Input: part model. Units: mm. Frame: model coordinates. Coordinates: 2 decimals unless noted, no trailing zeros. Loops run counter-clockwise (first coordinate to the right, second up) from the corner with the lowest first, then second, coordinate; pieces in that order, holes last. Notation, with made-up numbers: (46.5, 37.5) -> (92.5, 37.5) arc R24 ccw to (92.5, 62.5) -> close; hole circle Ø3 at (62, 78). An arc over 180 degrees is marked (long way). Answer as a JSON object with one key per item and string values.
from build123d import *
from OCP.BRepFilletAPI import BRepFilletAPI_MakeChamfer

# Parameters (mm, degrees)
BOSS_EXTRUDE1_DEPTH = 1.3
CUT_EXTRUDE1_DEPTH  = 7.730527468
CUT_EXTRUDE2_DEPTH  = 7.730527468
SKETCH4_W           = 6.4
SKETCH4_H           = 4.4
BOSS_EXTRUDE2_DEPTH = 0.3
SKETCH5_W           = 4.78
SKETCH5_H           = 1.3
BOSS_EXTRUDE3_DEPTH = 0.3
SKETCH6_W           = 4.78
SKETCH6_H           = 1.3
BOSS_EXTRUDE4_DEPTH = 0.3
DRAFT1_ANGLE        = 20
DRAFT2_ANGLE        = 20
HOLE1_D             = 0.497503641
HOLE1_DEPTH         = 0.2
CHAMFER1_SIZE       = 0.234692934
CHAMFER1_SIZE2      = 0.311889554
CHAMFER2_SIZE       = 0.311889554
CHAMFER2_SIZE2      = 0.234692934
FILLET1_R           = 0.5


with BuildPart() as part:
    # Sketch1 → Boss-Extrude1 (new body)
    with BuildSketch(Plane(origin=(0, 1.3, 0), x_dir=(1, 0, 0), z_dir=(0, 1, 0))):
        Polygon((3.5, 2.1), (0, 5.6), (-3.5, 2.1), (-3.5, -2.1), (0, -5.6), (3.5, -2.1), align=None)
    extrude(amount=-BOSS_EXTRUDE1_DEPTH)

    # Sketch2 → Cut-Extrude1 (cut, through all)
    with BuildSketch(Plane.XZ):
        Polygon((0, -5.6), (2.69, -2.91), (2.69, -2.2), (-2.69, -2.2), (-2.69, -2.91), align=None)
    extrude(amount=-CUT_EXTRUDE1_DEPTH, mode=Mode.SUBTRACT)

    # Sketch3 → Cut-Extrude2 (cut, through all)
    with BuildSketch(Plane.XZ):
        Polygon((2.69, 2.2), (2.69, 2.91), (0, 5.6), (-2.69, 2.91), (-2.69, 2.2), align=None)
    extrude(amount=-CUT_EXTRUDE2_DEPTH, mode=Mode.SUBTRACT)

    # Sketch4 → Boss-Extrude2 (add)
    with BuildSketch(Plane(origin=(0, 1.3, 0), x_dir=(-1, 0, 0), z_dir=(0, 1, 0))):
        Rectangle(SKETCH4_W, SKETCH4_H)
    extrude(amount=BOSS_EXTRUDE2_DEPTH)

    # Sketch5 → Boss-Extrude3 (add)
    with BuildSketch(Plane.XY.offset(2.2)):
        with Locations((0, 0.65)):
            Rectangle(SKETCH5_W, SKETCH5_H)
    extrude(amount=BOSS_EXTRUDE3_DEPTH)

    # Sketch6 → Boss-Extrude4 (add)
    with BuildSketch(Plane(origin=(0, 0, -2.2), x_dir=(-1, 0, 0), z_dir=(0, 0, -1))):
        with Locations((0, 0.65)):
            Rectangle(SKETCH6_W, SKETCH6_H)
    extrude(amount=BOSS_EXTRUDE4_DEPTH)

    # Draft1
    draft1_faces = [part.faces().sort_by_distance(p)[0] for p in [
        (-2.69, 0.65, -2.555),
        (-2.39, 0.65, -2.35),
        (2.39, 0.65, -2.35),
        (2.69, 0.65, -2.555),
    ]]
    draft(draft1_faces, Plane(origin=(2.69, 1.3, -2.2), x_dir=(-1, 0, 0), z_dir=(0, 0, -1)), DRAFT1_ANGLE)

    # Draft2
    draft2_faces = [part.faces().sort_by_distance(p)[0] for p in [
        (2.69, 0.65, 2.555),
        (2.39, 0.65, 2.35),
        (-2.39, 0.65, 2.35),
        (-2.69, 0.65, 2.555),
    ]]
    draft(draft2_faces, Plane(origin=(-2.69, 1.3, 2.2), x_dir=(1, 0, 0), z_dir=(0, 0, 1)), DRAFT2_ANGLE)

    # Hole1
    with Locations(Plane(origin=(0, 1.6, 0), x_dir=(1, 0, 0), z_dir=(0, 1, 0))):
        with Locations((-2.524000409, -1.40306368)):
            Hole(HOLE1_D / 2, depth=HOLE1_DEPTH)

    # Chamfer1: one chamfer whose edges measure the first distance from different faces: ONE call of the kernel's chamfer builder (chamfer() names one face for all edges)
    chamfer1_edges_1 = [part.edges().sort_by_distance(p)[0] for p in [
        (-2.879460781, 0.65, -2.720539219),
    ]]
    chamfer1_side_1 = [part.faces().sort_by_distance(p)[0] for p in [
        (-2.784730391, 0.65, -2.460269609),
    ]]
    chamfer1_edges_2 = [part.edges().sort_by_distance(p)[0] for p in [
        (2.879460781, 0.65, 2.720539219),
    ]]
    chamfer1_side_2 = [part.faces().sort_by_distance(p)[0] for p in [
        (2.784730391, 0.65, 2.460269609),
    ]]
    chamfer1 = BRepFilletAPI_MakeChamfer(part.part.solid().wrapped)
    for e in chamfer1_edges_1:
        chamfer1.Add(CHAMFER1_SIZE, CHAMFER1_SIZE2, e.wrapped, chamfer1_side_1[0].wrapped)  # the first distance lies on this face
    for e in chamfer1_edges_2:
        chamfer1.Add(CHAMFER1_SIZE, CHAMFER1_SIZE2, e.wrapped, chamfer1_side_2[0].wrapped)  # the first distance lies on this face
    add(Compound.cast(chamfer1.Shape()), mode=Mode.REPLACE)

    # Chamfer2: one chamfer whose edges measure the first distance from different faces: ONE call of the kernel's chamfer builder (chamfer() names one face for all edges)
    chamfer2_edges_1 = [part.edges().sort_by_distance(p)[0] for p in [
        (2.879460781, 0.65, -2.720539219),
    ]]
    chamfer2_side_1 = [part.faces().sort_by_distance(p)[0] for p in [
        (3.189730391, 0.65, -2.410269609),
    ]]
    chamfer2_edges_2 = [part.edges().sort_by_distance(p)[0] for p in [
        (-2.879460781, 0.65, 2.720539219),
    ]]
    chamfer2_side_2 = [part.faces().sort_by_distance(p)[0] for p in [
        (-3.189730391, 0.65, 2.410269609),
    ]]
    chamfer2 = BRepFilletAPI_MakeChamfer(part.part.solid().wrapped)
    for e in chamfer2_edges_1:
        chamfer2.Add(CHAMFER2_SIZE, CHAMFER2_SIZE2, e.wrapped, chamfer2_side_1[0].wrapped)  # the first distance lies on this face
    for e in chamfer2_edges_2:
        chamfer2.Add(CHAMFER2_SIZE, CHAMFER2_SIZE2, e.wrapped, chamfer2_side_2[0].wrapped)  # the first distance lies on this face
    add(Compound.cast(chamfer2.Shape()), mode=Mode.REPLACE)

    # Fillet1
    fillet1_edges = [part.edges().sort_by_distance(p)[0] for p in [
        (3.2, 1.45, -2.2),
        (-3.2, 1.45, -2.2),
        (-3.2, 1.45, 2.2),
        (3.2, 1.45, 2.2),
    ]]
    fillet(fillet1_edges, radius=FILLET1_R)


solid = part.part
1. Section query C-C (z = -1.6). Return loops of the section in (x, y).
Reply:
{"outline": "(-3.5, 0) -> (3.5, 0) -> (3.5, 1.3) -> (3.2, 1.3) -> (3.2, 1.6) -> (-3.2, 1.6) -> (-3.2, 1.3) -> (-3.5, 1.3) -> close"}
2. Line query: line 1 along Z through (x, y) = (-2.5, 1.45); line 2 along Y through (x, z) = (-1, 2.3); line 3 along X through (y, z) = (0.3, -2.25). Output: solid intervals per line, ascending.
Reply:
{"line 1": "z = -2.2 to 1.16, 1.65 to 2.2", "line 2": "y = 0 to 1.3", "line 3": "x = -3.35 to -2.71, -2.37 to 2.37, 2.71 to 3.35"}
3. Section query A-A (y = 0.45). Return loops of the section in (x, z).
Reply:
{"outline": "(-3.5, -2.1) -> (-3.1, -2.5) -> (-2.8, -2.5) -> (-2.69, -2.2) -> (-2.39, -2.2) -> (-2.28, -2.5) -> (2.28, -2.5) -> (2.39, -2.2) -> (2.69, -2.2) -> (2.8, -2.5) -> (3.1, -2.5) -> (3.5, -2.1) -> (3.5, 2.1) -> (3.1, 2.5) -> (2.8, 2.5) -> (2.69, 2.2) -> (2.39, 2.2) -> (2.28, 2.5) -> (-2.28, 2.5) -> (-2.39, 2.2) -> (-2.69, 2.2) -> (-2.8, 2.5) -> (-3.1, 2.5) -> (-3.5, 2.1) -> close"}
4. Section query B-B (x = 0). Return loops of the section in (y, z).
Reply:
{"outline": "(0, -2.5) -> (1.3, -2.5) -> (1.3, -2.2) -> (1.6, -2.2) -> (1.6, 2.2) -> (1.3, 2.2) -> (1.3, 2.5) -> (0, 2.5) -> close"}
